from build123d import *

# Parameters (mm, degrees)
F1_DEPTH = 12.7
F2_R     = 1.353731
F3_DEPTH = 50.8


with BuildPart() as f1:
    # F0 (on Front) → F1 (new body)
    with BuildSketch(Plane.XZ):
        Polygon((38.97683, 29.645005), (-18.17317, 29.645005), (-18.17317, 23.295005), (10.40183, 23.295005), (38.97683, 23.295005), align=None)
        Polygon((67.55183, 23.295005), (38.97683, 23.295005), (10.40183, 23.295005), (10.40183, 17.107827), (67.55183, 17.107827), align=None)
    extrude(amount=F1_DEPTH)

    # F2 (on Top) → F3 (cut)
    with BuildSketch(Plane.XY):
        with Locations((-11.172788, -6.245584)):
            Circle(F2_R)
    extrude(amount=F3_DEPTH, mode=Mode.SUBTRACT)


solid = f1.part
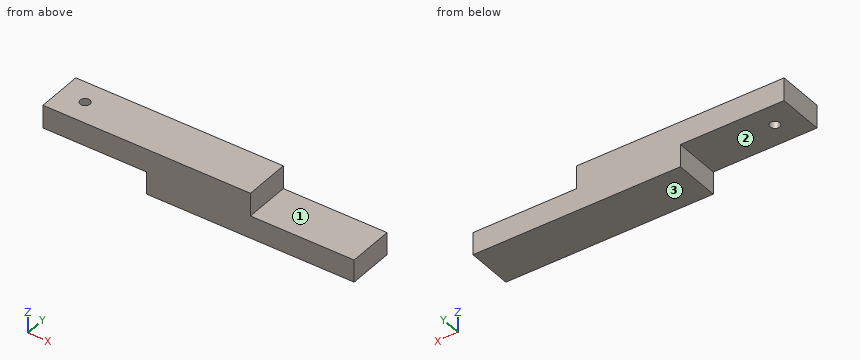
Input: part model. Units: mm. Frame: model coordinates. Face numbers are marked on the shaded views. A direction names the side the tool comes from. Coordinates: 2 decimals unless noted, no trailing zeros. Loops run counter-clockwise (first coordinate to the right, second up) from the corner with the lowest first, then second, coordinate; pieces in that order, holes last. Notation, with made-up numbers: (28.25, 23.5) -> (44.25, 23.5) arc R13 ccw to (44.25, 28.5) -> close; hole circle Ø7 at (17, -9). An arc over 180 degrees is marked (long way). Write item = value, one per line. Start each with the question number.
Item 1: Reachability of the marked faces 1, 2 and 3 from +Z, -Z, +X, -X, +Y, -Y: full face, straight path, thin tool, end or side. Return the list, or none.
Item 2: First-contact query: P1, Ø5, axis at y = -6, z = 19, coming from the -X side; P2, Ø6.5, axis at x = -3.5, y = -6.5, coming from the -Z side (3 decimals); P3, Ø1, axis at y = -10.5, z = 24, coming from the +X side; P4, Ø2, axis at x = -11.17, y = -6.25, coming from the +Z side. Flat tips, straight axial feed; report the tip coordinate or a pass-through.
Item 3: Material intervals for line 1 (X direction, y = -10.5, z = 22.5); line 2 (X direction, y = -4.75, z = 27.75); line 3 (Z direction, x = 9, y = -8.25) (3 decimals), sorted ascending.
Item 4: Cut plane D-D, the plane x = 49. Return loops of the section in (y, z) (3 decimals).
Item 5: Cut plane B-B, the plane z = 27.5. Return loops of the section in (x, y).
Item 6: Cut plane C-C, the plane z = 18. Return loops of the section in (x, y).
Item 7: Cut plane A-A, the plane y = -10.25. Return loops of the section in (x, z) (3 decimals), plus the area to 4 significant figures.
Ans:
q1.face_1 = +Z, +X, +Y, -Y
q1.face_2 = -Z, -X, +Y, -Y
q1.face_3 = -Z, +X, -X, +Y, -Y
q2.P1 = 10.4
q2.P2 = 23.295
q2.P3 = 38.98
q2.P4 = through
q3.line_1 = 10.4 to 67.55
q3.line_2 = -18.17 to 38.98
q3.line_3 = 23.295 to 29.645
q4.outline = (-12.7, 17.108) -> (0, 17.108) -> (0, 23.295) -> (-12.7, 23.295) -> close
q5.outline = (-18.17, -12.7) -> (38.98, -12.7) -> (38.98, 0) -> (-18.17, 0) -> close; hole circle Ø2.71 at (-11.17, -6.25)
q6.outline = (10.4, -12.7) -> (67.55, -12.7) -> (67.55, 0) -> (10.4, 0) -> close
q7.outline = (-18.173, 23.295) -> (10.402, 23.295) -> (10.402, 17.108) -> (67.552, 17.108) -> (67.552, 23.295) -> (38.977, 23.295) -> (38.977, 29.645) -> (-18.173, 29.645) -> close
q7.area = 716.5 mm²
